Here's how the part is built. I have some questions about the finished solid (model axes, mm). Face numbers are marked on the shaded views. Coordinates: 2 decimals unless noted, no trailing zeros. Write each loop counter-clockwise with the first axis right and the second up, starting at its lowest first coordinate (ties: lowest second). Pieces come first, ordered by that corner, then holes. Notation, with made-up numbers: (-7, 22) - (6, 22) arc R24 ccw to (6, 40) - close; hole circle Ø1 at (89.25, -27.5). An arc over 180 degrees is marked (long way). Answer in a Markdown table with one row per item. Add a question column.
Item 1: We'd pull the mould along Y, two halves only. Please class the marked faces 1 and 2: +Y half, -Y half, draft (parallel to the pull), parting line (faces both ways), or undercut.
Item 2: I'm going to push flat-ended pins straight in: pin 1 (1.9 mm diameter, centred on x = 58, y = 2.5, fed in from -Z); pin 2 (3 mm diameter, centred on y = 4.5, z = 1.5, fed in from -X) (3 decimals); pin 3 (3 mm diameter, centred on x = -47.5, y = 2, fed in from +Z). Where does each tip first touch, or does it pass through?
Item 3: If I drill on probe 1 along X at (y, z) = (1.5, 0) (3 decimals); probe 2 along Z at (x, y) = (45.5, 1) (3 decimals); probe 3 along Z at (x, y) = (54.5, 1.5) (3 decimals), over which ranges is the centre line in solid material (lowest first)? Write a range as from..to.
Item 4: Imagine slicing it at D-D (x = 18). Please give me the cut outline in (y, z).
Item 5: Imagine slicing it at C-C (y = 1). Please give me the cut outline in (x, z) (3 decimals).
Item 6: Imagine slicing it at A-A (z = 0). Please give me the cut outline in (x, y) (3 decimals).
Item 7: Imagine slicing it at B-B (x = 0). Please give me the cut outline in (y, z) (3 decimals), plus the area to 3 significant figures.
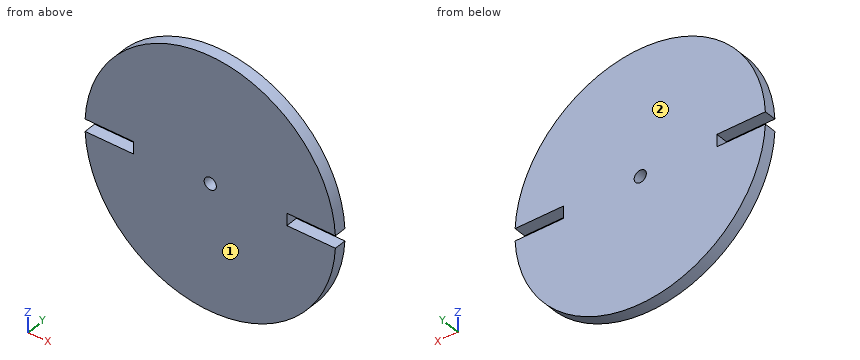
from build123d import *

# Parameters (mm, degrees)
SKETCH1_R           = 65.405
BOSS_EXTRUDE1_DEPTH = 6.35
SKETCH2_W           = 50.8
SKETCH2_H           = 6.35
CUT_EXTRUDE1_DEPTH  = 6.35
SKETCH7_R           = 3.175
CUT_EXTRUDE2_DEPTH  = 7.35


with BuildPart() as part:
    # Sketch1 → Boss-Extrude1 (new body)
    with BuildSketch(Plane(origin=(0, 0, 0), x_dir=(1, 0, 0), z_dir=(0, 1, 0))):
        Circle(SKETCH1_R)
    extrude(amount=BOSS_EXTRUDE1_DEPTH)

    # Sketch2 → Cut-Extrude1 (cut)
    with BuildSketch(Plane(origin=(0, 6.35, 0), x_dir=(1, 0, 0), z_dir=(0, 1, 0))):
        with Locations((-65.405, 0)):
            Rectangle(SKETCH2_W, SKETCH2_H)
        with Locations((65.405, 0)):
            Rectangle(SKETCH2_W, SKETCH2_H)
    extrude(amount=-CUT_EXTRUDE1_DEPTH, mode=Mode.SUBTRACT)

    # Sketch7 → Cut-Extrude2 (cut, through all)
    with BuildSketch(Plane(origin=(0, 6.35, 0), x_dir=(1, 0, 0), z_dir=(0, 1, 0))):
        Circle(SKETCH7_R)
    extrude(amount=-CUT_EXTRUDE2_DEPTH, mode=Mode.SUBTRACT)


solid = part.part
Here are the results:
| question | item | result |
|---|---|---|
| 1 | face 1 | -Y half |
| 1 | face 2 | +Y half |
| 2 | pin 1 | stops at z = -31.99 |
| 2 | pin 2 | stops at x = -40.005 |
| 2 | pin 3 | stops at z = 46.5 |
| 3 | probe 1 | x = -40.005..-3.175, 3.175..40.005 |
| 3 | probe 2 | z = -46.985..-3.175, 3.175..46.985 |
| 3 | probe 3 | z = -36.16..-3.175, 3.175..36.16 |
| 4 | outline | (0, -62.88) - (6.35, -62.88) - (6.35, 62.88) - (0, 62.88) - close |
| 5 | outline | (-65.328, -3.175) arc R65.405 ccw to (65.328, -3.175) - (40.005, -3.175) - (40.005, 3.175) - (65.328, 3.175) arc R65.405 ccw to (-65.328, 3.175) - (-40.005, 3.175) - (-40.005, -3.175) - close; hole circle Ø6.35 at (0, 0) |
| 6 | outline | (-40.005, 0) - (-3.175, 0) - (-3.175, 6.35) - (-40.005, 6.35) - close; (3.175, 0) - (40.005, 0) - (40.005, 6.35) - (3.175, 6.35) - close |
| 7 | outline | (0, -65.405) - (6.35, -65.405) - (6.35, -3.175) - (0, -3.175) - close; (0, 3.175) - (6.35, 3.175) - (6.35, 65.405) - (0, 65.405) - close |
| 7 | area | 790 mm2 |
